Autodesk Inventor part; units mm, degrees
ref_plane "YZ Plane" through (0, 0, 0) normal (1, 0, 0) x (0, 1, 0)
ref_plane "XZ Plane" through (0, 0, 0) normal (0, 1, 0) x (-1, 0, 0)
ref_plane "XY Plane" through (0, 0, 0) normal (0, 0, 1) x (1, 0, 0)
sketch "스케치1" plane through (0, 0, 0) normal (0, 0, 1) x (1, 0, 0)
  line L0 (0, 0) -> (9, 0)
  line L1 (9, 0) -> (9, 10.8)
  line L2 (9, 10.8) -> (0, 10.8)
  line L3 (0, 10.8) -> (0, 0)
  line L4 (-1.2, 12) -> (10.2, 12)
  line L5 (10.2, 12) -> (10.2, -1.2)
  line L6 (10.2, -1.2) -> (-1.2, -1.2)
  line L7 (-1.2, -1.2) -> (-1.2, 12)
  line L8 (0, 0) -> (0, -1.2)
  line L9 (9, 0) -> (9, -1.2)
  line L10 (0, 0) -> (-1.2, 0)
  line L11 (9, 0) -> (10.2, 0)
  arc A0 (-1.2, 12) -> (-1.2, -1.2) centre (3.7811, 5.4) ccw
  arc A1 (0, 10.8) -> (0, 0) centre (3.7811, 5.4) ccw
  line L12 (-1.2, 10.4) -> (0, 10.4) construction
  line L13 (0, 10.4) -> (0, 0.4) construction
  line L14 (0, 0.4) -> (-1.2, 0.4) construction
  line L15 (-1.2, 0.4) -> (-1.2, 10.4) construction
  point P0 (0, 5.4)
  dimension "d0" = 9
  dimension "d1" = 10.8
  dimension "d2" = 1.2
  dimension "d35" = 10
  dimension "d36" = 110
extrude "돌출1" add sketch "스케치1" along normal blind 20 contours L8 L6 L7 L10 | L10 L7 A1 | L11 L5 L6 L9 | L1 L2 A1 L7 L4 L5 L11 | L7 A0 A1
sketch "스케치5" plane through (0, 10.8, 0) normal (0, -1, 0) x (1, 0, 0)
  line L0 (0, 0) -> (9, 0)
  line L1 (9, 0) -> (9, 20)
  line L2 (0, 20) -> (9, 20)
  line L3 (0, 0) -> (0, 20)
  line L4 (9, 17.5) -> (7, 17.5)
  line L5 (7, 17.5) -> (7, 20)
  line L6 (10.2, 20) -> (-1.2, 20)
  point P0 (0, 0)
  point P1 (8.2, 20)
  point P2 (-0.4776, 20)
  dimension "d21" = 2.5
  dimension "d22" = 2
extrude "돌출5" add sketch "스케치5" along normal blind 5 contours L4 L5 L2 L1
sketch "스케치8" plane through (0, -1.2, 0) normal (1, 0, 0) x (0, 0, -1)
  line L0 (0, 0) -> (-20, 0)
  line L1 (0, 0) -> (0, 1.2)
  line L2 (0, 0) -> (-20, 0)
  line L3 (-5, 0) -> (-5.8, 0)
  line L4 (-5.8, 0) -> (-5.8, 8)
  line L5 (-5.8, 8) -> (-5, 8)
  line L6 (-5, 8) -> (-5, 0)
  point P0 (-18.5, 0)
  point P1 (-5.8, 0)
  point P2 (-5, 0)
  dimension "d37" = 5
  dimension "d38" = 0.8
  dimension "d39" = 8
extrude "돌출7" cut sketch "스케치8" against normal through all
sketch "스케치13" plane through (0, 0, 20) normal (0, 0, 1) x (1, 0, 0)
  line L0 (0, 10.8) -> (7, 10.8)
  line L1 (9, 5.8) -> (9, -1.2)
  line L2 (9, -1.2) -> (10.2, -1.2)
  line L3 (10.2, -1.2) -> (10.2, 12)
  line L4 (10.2, 12) -> (-1.2, 12)
  arc A0 (-1.2, 12) -> (-1.2, -1.2) centre (3.7811, 5.4) ccw
  line L5 (-1.2, -1.2) -> (0, -1.2)
  line L6 (0, -1.2) -> (0, 0)
  arc A1 (0, 10.8) -> (0, 0) centre (3.7811, 5.4) ccw
  line L7 (0, 10.8) -> (9, 10.8)
  line L8 (7, 10.8) -> (9, 10.8)
  line L9 (9, 10.8) -> (9, 5.8)
extrude "돌출11" add sketch "스케치13" along normal blind 5.5
sketch "스케치14" plane through (0, 0, 25.5) normal (0, 0, 1) x (1, 0, 0)
  line L0 (10.2, -1.2) -> (10.2, 12)
  line L1 (10.2, 12) -> (-1.2, 12)
  arc A0 (-1.2, 12) -> (-1.2, -1.2) centre (3.7811, 5.4) ccw
  line L2 (-1.2, -1.2) -> (0, -1.2)
  line L3 (0, -1.2) -> (0, 0)
  arc A1 (0, 10.8) -> (0, 0) centre (3.7811, 5.4) ccw
  line L4 (0, 10.8) -> (9, 10.8)
  arc A2 (-0.8195, 11.55) -> (-0.8195, -0.75) centre (4.7076, 5.4) ccw
  line L5 (-0.8195, 11.55) -> (10.2, 11.55)
  line L6 (10.2, -1.2) -> (10.2, 12)
  line L7 (-0.8195, -0.75) -> (0, -0.75)
  dimension "d53" = 0.75
  dimension "d55" = 0.75
  dimension "d56" = 0.75
extrude "돌출12" add sketch "스케치14" along normal blind 1
sketch "스케치15" plane through (0, 0, 26.5) normal (0, 0, 1) x (1, 0, 0)
  line L0 (10.2, 11.55) -> (10.2, 12)
  line L1 (10.2, 12) -> (-1.2, 12)
  arc A0 (-1.2, 12) -> (-1.2, -1.2) centre (3.7811, 5.4) ccw
  line L2 (-1.2, -1.2) -> (0, -1.2)
  line L3 (0, -1.2) -> (0, -0.75)
  line L4 (10.2, 11.55) -> (-0.8195, 11.55)
  arc A1 (-0.8195, 11.55) -> (-0.8195, -0.75) centre (4.7076, 5.4) ccw
  line L5 (-0.8195, -0.75) -> (0, -0.75)
  line L6 (0, -0.75) -> (0, 0)
  arc A2 (0, 10.8) -> (0, 0) centre (3.7811, 5.4) ccw
  line L7 (0, 10.8) -> (9, 10.8)
  line L8 (9, 10.8) -> (9, -1.2)
  line L9 (9, -1.2) -> (10.2, -1.2)
  line L10 (10.2, -1.2) -> (10.2, 11.55)
  line L11 (9, 10.8) -> (10.2, 10.8)
extrude "돌출13" add sketch "스케치15" along normal blind 1 contours L4 A1 L5 L3 L2 A0 L1 L0 | L10 L11 L7 A2 L6 L5 A1 L4
fillet "모깎기2" radius 2 2 edges at (10.2, 12, 13.75) (-1.2, 12, 13.75)
equation "\"d56\" = d55"
properties part number "_3D 인쇄"
The listing builds one solid part. Answer for the finished solid, in the listing's coordinates (mm). A direction names the side the tool comes from. Coordinates: 2 decimals unless noted, no trailing zeros. Order: outer loops, then holes, each group sorted by start corner. A loop starts at its lowest first (then second) coordinate and runs counter-clockwise, first axis right, second up.
Q1. Which of the six approach directions +Z, -Z, +X, -X, +Y, -Y give full straight-line access (tool end or side, diameter ignored) to faces 4 (the face through (8, 8, 17.5)), 5 (the face through (7, 8, 19)), 6 (the face through (5, 10.8, 27))?
Q2. For a pull along Y with two mould halves and no side action, classify faces 1 (the face through (-0.4, -0.75, 26)), 2 (the face through (-3, 3, 5)), 3 (the face through (-1, -1.2, 2)) as pulls with the +Y half, pulls with the -Y half, needs draft (parallel to the pull), parting line crosses it, or undercut.
Q3. Consider line 1 (Z direction, x = 1, y = 11); line 2 (Y direction, x = 7, z = 4.25); line 3 (Y direction, x = 7.5, z = 26). Determine where each line is inside the solid, lowest interval first.
Q4. Given P1, Ø2, axis at x = 7.5, y = 8, coming from the +Z side; P2, Ø1.2, axis at y = 9, z = 19, coming from the -X side; P3, Ø2, axis at x = 0, y = 6.5, coming from the -Z side; P4, Ø0.8, axis at x = 3.5, z = 27, coming from the -Y side, each flat-ended and moving along its own axis, determine where each tip first touches the part or whether it passes through.
Q5. A cutting plane is placed at C-C, the plane z = 18.75. Write down the section's boundary in (x, y).
Q6. A cutting plane is placed at A-A, the plane y = 3.5. Write down the section's boundary in (x, z).
Q7. A cutting plane is placed at D-D, the plane y = 7.75. Write down the section's boundary in (x, z).
Q8. A cutting plane is placed at B-B, the plane x = 7.5. Write down the section's boundary in (y, z).
Answers follow:
1. face 4: -Z, -Y
1. face 5: +Z, -Z, -Y
1. face 6: +Z, +X, -Y
2. face 1: undercut
2. face 2: needs draft
2. face 3: pulls with the -Y half
3. line 1: z = 0 to 25.5, 26.5 to 27.5
3. line 2: y = 10.8 to 12
3. line 3: y = 11.55 to 12
4. P1: stops at z = 20
4. P2: stops at x = -3.92
4. P3: passes through
4. P4: stops at y = 10.8
5. outline: (-1.84, 11.47) arc R8.27 ccw to (-1.2, -1.2) - (0, -1.2) - (0, 0) arc R6.59 cw to (0, 10.8) - (7, 10.8) - (7, 5.8) - (9, 5.8) - (9, -1.2) - (10.2, -1.2) - (10.2, 10) arc R2 ccw to (8.2, 12) - (-0.48, 12) arc R2 ccw to start
6. outline: (-4.27, 0) - (-2.53, 0) - (-2.53, 5) - (-4.27, 5) - close; (-4.27, 5.8) - (-2.53, 5.8) - (-2.53, 25.5) - (-3.34, 25.5) - (-3.34, 26.5) - (-2.53, 26.5) - (-2.53, 27.5) - (-4.27, 27.5) - close; (9, 0) - (10.2, 0) - (10.2, 25.5) - (9, 25.5) - close
7. outline: (-4.15, 0) - (-2.38, 0) - (-2.38, 25.5) - (-3.22, 25.5) - (-3.22, 26.5) - (-2.38, 26.5) - (-2.38, 27.5) - (-4.15, 27.5) - close; (7, 17.5) - (9, 17.5) - (9, 0) - (10.2, 0) - (10.2, 25.5) - (9, 25.5) - (9, 20) - (7, 20) - close
8. outline: (5.8, 17.5) - (10.8, 17.5) - (10.8, 0) - (12, 0) - (12, 27.5) - (10.8, 27.5) - (10.8, 26.5) - (11.55, 26.5) - (11.55, 25.5) - (10.8, 25.5) - (10.8, 20) - (5.8, 20) - close
